Geometry: final body of the model. Coordinates: model frame, mm. Face numbers are marked on the shaded views. A direction names the side the tool comes from. Round coordinates to 2 decimals unless told otherwise and drop trailing zeros. Order: outer loops, then holes, each group sorted by start corner. A loop starts at its lowest first (then second) coordinate and runs counter-clockwise, first axis right, second up. Notation, with made-up numbers: M -31,-36 L 13,-36 A8 ccw 13,-27 Z; hole C 29.5,-2 d3. An arc over 180 degrees is marked long. Put each result on its own line as item: value. Start each with the question number.
1) Material intervals for probe 1 along Y at (x, z) = (-4, -32); probe 2 along Y at (x, z) = (5, 4.5), sorted ascending. Write a range as [from, to].
2) Section B-B, the plane z = 10. Return loops of the section in (x, y).
3) First-contact query: P1, Ø5, axis at y = 25, z = 10, coming from the +X side; P2, Ø12.5, axis at x = -3, y = -3, coming from the +Z side; P3, Ø8, axis at y = -4.5, z = -12.5, coming from the -X side; P4, Ø10, axis at y = 12.5, z = -49, coming from the +X side. Flat tips, straight axial feed; report the tip coordinate or a pass-through.
4) Draft query along Z for the marked faces 1, 2, 3 and 4. Return one class per face: pulls with the +Z half, pulls with the -Z half, needs draft (parallel to the pull), parting line crosses it, or undercut.
5) Section A-A, the plane y = 25. Return loops of the section in (x, z), then the cut area to 3 significant figures.
6) Access query for the marked faces 5 and 6. Directions: +Z, -Z, +X, -X, +Y, -Y. A direction counts if a zero-diameter tool reaches every point of the face in a straight line with its end or side. Return the directions, or none.
from build123d import *

# Parameters (mm, degrees)
EXTRUDE_1_DEPTH          = 5
SKETCH_3_R               = 1.5
EXTRUDE_2_DEPTH          = 4
CUT_EXTRUDE_1_DEPTH      = 112.469065397
PATTERN_CIRCULAR_1_COUNT = 3
FILLET_1_R               = 3
FILLET_2_R               = 5


with BuildPart() as part:
    # 草图1 → 旋转1 (revolve)
    with BuildSketch(Plane(origin=(0, 0, 0), x_dir=(0, 0, -1), z_dir=(1, 0, 0)), mode=Mode.PRIVATE) as revolve_1_sk:
        Polygon((0, 0), (0, 12.5), (3, 12.5), (10.5, 5), (79, 5), (79, 8), (82, 8), (82, 5), (102, 5), (102, 8), (105, 8), (105, 0), align=None)
    revolve(revolve_1_sk.sketch.rotate(Axis((0, 0, 0), (0, 0, -1)), 90), axis=Axis((0, 0, 0), (0, 0, -1)))

    # 草图2 → 凸台-拉伸1 (add)
    with BuildSketch(Plane.XY):
        Polygon((-4, 25), (4, 25), (4, 18.07179677), (17.650635095, -5.57179677), (23.650635095, -9.035898385), (19.650635095, -15.964101615), (13.650635095, -12.5), (-13.650635095, -12.5), (-19.650635095, -15.964101615), (-23.650635095, -9.035898385), (-17.650635095, -5.57179677), (-4, 18.07179677), align=None)
    extrude(amount=EXTRUDE_1_DEPTH)

    # 草图3 → 凸台-拉伸2 (add, symmetric)
    with BuildSketch(Plane(origin=(0, 0, 0), x_dir=(0, 0, -1), z_dir=(1, 0, 0))):
        with BuildLine():
            Line((-5, 7.5), (-13.510549927, 23.082700021))
            ThreePointArc((-13.510549927, 23.082700021), (-12.95059807, 27.700735275), (-8.4, 28.666060556))
            Line((-8.4, 28.666060556), (0, 25))
            Line((0, 25), (-5, 25))
            Line((-5, 25), (-5, 7.5))
        make_face()
        with Locations((-10, 25)):
            Circle(SKETCH_3_R, mode=Mode.SUBTRACT)
    extrude_2 = extrude(amount=EXTRUDE_2_DEPTH, both=True)

    # 草图5 → 切除-拉伸1 (cut, symmetric)
    with BuildSketch(Plane(origin=(0, 0, 0), x_dir=(0, 0, -1), z_dir=(1, 0, 0))):
        Polygon((0, 20), (-6.415605973, 27.8), (0, 25), align=None)
    cut_extrude_1 = extrude(amount=CUT_EXTRUDE_1_DEPTH, both=True, mode=Mode.SUBTRACT)

    # 阵列(圆周)1: 凸台-拉伸2, 切除-拉伸1 ×3 about axis
    pattern_circular_1_axis = Axis((0, 0, 0), (0, 0, 1))
    add([extrude_2.rotate(pattern_circular_1_axis, i * 360 / PATTERN_CIRCULAR_1_COUNT) for i in range(1, PATTERN_CIRCULAR_1_COUNT)])
    add([cut_extrude_1.rotate(pattern_circular_1_axis, i * 360 / PATTERN_CIRCULAR_1_COUNT) for i in range(1, PATTERN_CIRCULAR_1_COUNT)], mode=Mode.SUBTRACT)

    # 圆角1
    # the kernel refuses this fillet: 3 mm, written as the material it adds along each edge
    with BuildSketch(Plane(origin=(20.145825623, -16.25, 5), x_dir=(0, 0, 1), z_dir=(-0.8660254037844384, 0.5000000000000004, 0))) as fillet_1_piece_1_section:
        with BuildLine():
            CenterArc((FILLET_1_R, -FILLET_1_R), FILLET_1_R, 90, 90)
            Line((0, -FILLET_1_R), (0, 0))
            Line((0, 0), (FILLET_1_R, 0))
        make_face()
    fillet_1_piece_1 = extrude(amount=25.57179677, mode=Mode.PRIVATE)
    fillet_1_piece_1 = split(fillet_1_piece_1, bisect_by=Plane(origin=(20.145825623, -12.5, 5), z_dir=(0, 1, 0)), keep=Keep.TOP, mode=Mode.PRIVATE)
    fillet_1_piece_1 = split(fillet_1_piece_1, bisect_by=Plane(origin=(16.550053856, -14.173980202, 12.602327469), z_dir=(0.4151076221534179, -0.23966249739294157, -0.877637481750588)), keep=Keep.TOP, mode=Mode.PRIVATE)
    add(fillet_1_piece_1)
    with BuildSketch(Plane(origin=(24.145825623, -9.32179677, 5), x_dir=(0, 0, 1), z_dir=(-0.8660254037844384, 0.5000000000000004, 0))) as fillet_1_piece_2_section:
        with BuildLine():
            CenterArc((FILLET_1_R, FILLET_1_R), FILLET_1_R, 180, 90)
            Line((0, FILLET_1_R), (0, 0))
            Line((0, 0), (FILLET_1_R, 0))
        make_face()
    fillet_1_piece_2 = extrude(amount=25.57179677, mode=Mode.PRIVATE)
    fillet_1_piece_2 = split(fillet_1_piece_2, bisect_by=Plane(origin=(20.550053856, -7.245776972, 12.602327469), z_dir=(0.4151076221534179, -0.23966249739294157, -0.877637481750588)), keep=Keep.TOP, mode=Mode.PRIVATE)
    fillet_1_piece_2 = split(fillet_1_piece_2, bisect_by=Plane(origin=(20.898230359, -11.19679677, 5), z_dir=(-0.8660254037844386, -0.5000000000000001, 0)), keep=Keep.TOP, mode=Mode.PRIVATE)
    add(fillet_1_piece_2)
    with BuildSketch(Plane(origin=(4, 25.57179677, 5), x_dir=(0, 0, 1), z_dir=(0, -1, 0))) as fillet_1_piece_3_section:
        with BuildLine():
            CenterArc((FILLET_1_R, -FILLET_1_R), FILLET_1_R, 90, 90)
            Line((0, -FILLET_1_R), (0, 0))
            Line((0, 0), (FILLET_1_R, 0))
        make_face()
    fillet_1_piece_3 = extrude(amount=25.57179677, mode=Mode.PRIVATE)
    fillet_1_piece_3 = split(fillet_1_piece_3, bisect_by=Plane(origin=(0.752404736, 23.69679677, 5), z_dir=(-0.8660254037844386, -0.5000000000000001, 0)), keep=Keep.TOP, mode=Mode.PRIVATE)
    fillet_1_piece_3 = split(fillet_1_piece_3, bisect_by=Plane(origin=(4, 21.419757175, 12.602327469), z_dir=(0, 0.4793249947858827, -0.877637481750588)), keep=Keep.TOP, mode=Mode.PRIVATE)
    add(fillet_1_piece_3)
    with BuildSketch(Plane(origin=(-4, 25.57179677, 5), x_dir=(0, 0, 1), z_dir=(0, -1, 0))) as fillet_1_piece_4_section:
        with BuildLine():
            CenterArc((FILLET_1_R, FILLET_1_R), FILLET_1_R, 180, 90)
            Line((0, FILLET_1_R), (0, 0))
            Line((0, 0), (FILLET_1_R, 0))
        make_face()
    fillet_1_piece_4 = extrude(amount=25.57179677, mode=Mode.PRIVATE)
    fillet_1_piece_4 = split(fillet_1_piece_4, bisect_by=Plane(origin=(-0.752404736, 23.69679677, 5), z_dir=(0.8660254037844388, -0.4999999999999999, 0)), keep=Keep.TOP, mode=Mode.PRIVATE)
    fillet_1_piece_4 = split(fillet_1_piece_4, bisect_by=Plane(origin=(-4, 21.419757175, 12.602327469), z_dir=(0, 0.4793249947858827, -0.877637481750588)), keep=Keep.TOP, mode=Mode.PRIVATE)
    add(fillet_1_piece_4)
    with BuildSketch(Plane(origin=(-24.145825623, -9.32179677, 5), x_dir=(0, 0, 1), z_dir=(0.8660254037844388, 0.49999999999999983, 0))) as fillet_1_piece_5_section:
        with BuildLine():
            CenterArc((FILLET_1_R, -FILLET_1_R), FILLET_1_R, 90, 90)
            Line((0, -FILLET_1_R), (0, 0))
            Line((0, 0), (FILLET_1_R, 0))
        make_face()
    fillet_1_piece_5 = extrude(amount=25.57179677, mode=Mode.PRIVATE)
    fillet_1_piece_5 = split(fillet_1_piece_5, bisect_by=Plane(origin=(-20.898230359, -11.19679677, 5), z_dir=(0.8660254037844388, -0.4999999999999999, 0)), keep=Keep.TOP, mode=Mode.PRIVATE)
    fillet_1_piece_5 = split(fillet_1_piece_5, bisect_by=Plane(origin=(-20.550053856, -7.245776972, 12.602327469), z_dir=(-0.4151076221534181, -0.23966249739294126, -0.8776374817505879)), keep=Keep.TOP, mode=Mode.PRIVATE)
    add(fillet_1_piece_5)
    with BuildSketch(Plane(origin=(-20.145825623, -16.25, 5), x_dir=(0, 0, 1), z_dir=(0.8660254037844388, 0.49999999999999983, 0))) as fillet_1_piece_6_section:
        with BuildLine():
            CenterArc((FILLET_1_R, FILLET_1_R), FILLET_1_R, 180, 90)
            Line((0, FILLET_1_R), (0, 0))
            Line((0, 0), (FILLET_1_R, 0))
        make_face()
    fillet_1_piece_6 = extrude(amount=25.57179677, mode=Mode.PRIVATE)
    fillet_1_piece_6 = split(fillet_1_piece_6, bisect_by=Plane(origin=(-20.145825623, -12.5, 5), z_dir=(0, 1, 0)), keep=Keep.TOP, mode=Mode.PRIVATE)
    fillet_1_piece_6 = split(fillet_1_piece_6, bisect_by=Plane(origin=(-16.550053856, -14.173980202, 12.602327469), z_dir=(-0.4151076221534181, -0.23966249739294126, -0.8776374817505879)), keep=Keep.TOP, mode=Mode.PRIVATE)
    add(fillet_1_piece_6)

    # 圆角2
    # the kernel refuses this fillet: 5 mm, written as the material it adds along each edge
    with BuildSketch(Plane(origin=(0, 0, 0), x_dir=(-0.8660253934759007, 0.5000000178549112, 0), z_dir=(-0.5000000178549112, -0.8660253934759007, 0))) as fillet_2_piece_1_section:
        with BuildLine():
            CenterArc((17.082575695, 5), FILLET_2_R, 203.578178478, 66.421821522)
            Line((17.082575695, 0), (12.5, 0))
            Line((12.5, 0), (12.5, 3))
        make_face()
    fillet_2_piece_1 = revolve(axis=Axis((0, 0, 0), (0, 0, -1)), revolution_arc=119.999998782, mode=Mode.PRIVATE)
    fillet_2_piece_1 = split(fillet_2_piece_1, bisect_by=Plane(origin=(-10.825317547, 6.25, 0), z_dir=(0.866025403784329, -0.50000000000019, 0)), keep=Keep.TOP, mode=Mode.PRIVATE)
    fillet_2_piece_1 = split(fillet_2_piece_1, bisect_by=Plane(origin=(10.825317547, 6.25, 0), z_dir=(-0.866025403784329, -0.50000000000019, 0)), keep=Keep.TOP, mode=Mode.PRIVATE)
    add(fillet_2_piece_1)
    with BuildSketch(Plane(origin=(0, 0, 0), x_dir=(3.791753972085742e-09, -1.0, 0), z_dir=(1.0, 3.791753972085742e-09, 0))) as fillet_2_piece_2_section:
        with BuildLine():
            CenterArc((17.082575695, 5), FILLET_2_R, 203.578178478, 66.421821522)
            Line((12.5, 3), (12.5, 0))
            Line((12.5, 0), (17.082575695, 0))
        make_face()
    fillet_2_piece_2 = revolve(axis=Axis((0, 0, 0), (0, 0, -1)), revolution_arc=120.000001399, mode=Mode.PRIVATE)
    fillet_2_piece_2 = split(fillet_2_piece_2, bisect_by=Plane(origin=(-10.825317547, 6.25, 0), z_dir=(0.866025403784329, -0.50000000000019, 0)), keep=Keep.TOP, mode=Mode.PRIVATE)
    fillet_2_piece_2 = split(fillet_2_piece_2, bisect_by=Plane(origin=(0, -12.5, 0), z_dir=(0, 1, 0)), keep=Keep.TOP, mode=Mode.PRIVATE)
    add(fillet_2_piece_2)
    with BuildSketch(Plane(origin=(0, 0, 0), x_dir=(1, 0, 0), z_dir=(0, 1, 0))) as fillet_2_piece_3_section:
        with BuildLine():
            CenterArc((17.082575695, 5), FILLET_2_R, 203.578178478, 66.421821522)
            Line((17.082575695, 0), (12.5, 0))
            Line((12.5, 0), (12.5, 3))
        make_face()
    fillet_2_piece_3 = revolve(axis=Axis((0, 0, 0), (0, 0, -1)), revolution_arc=89.999999783, mode=Mode.PRIVATE)
    fillet_2_piece_3 = split(fillet_2_piece_3, bisect_by=Plane(origin=(10.825317547, 6.25, 0), z_dir=(-0.866025403784329, -0.50000000000019, 0)), keep=Keep.TOP, mode=Mode.PRIVATE)
    fillet_2_piece_3 = split(fillet_2_piece_3, bisect_by=Plane(origin=(0, -12.5, 0), z_dir=(0, 1, 0)), keep=Keep.TOP, mode=Mode.PRIVATE)
    add(fillet_2_piece_3)
    with BuildSketch(Plane(origin=(0, 0, 0), x_dir=(0.8660254034677206, 0.5000000005485719, 0), z_dir=(-0.5000000005485719, 0.8660254034677206, 0))) as fillet_2_piece_4_section:
        with BuildLine():
            CenterArc((17.082575695, 5), FILLET_2_R, 203.578178478, 66.421821522)
            Line((17.082575695, 0), (12.5, 0))
            Line((12.5, 0), (12.5, 3))
        make_face()
    fillet_2_piece_4 = revolve(axis=Axis((0, 0, 0), (0, 0, -1)), revolution_arc=30.000000036, mode=Mode.PRIVATE)
    fillet_2_piece_4 = split(fillet_2_piece_4, bisect_by=Plane(origin=(10.825317547, 6.25, 0), z_dir=(-0.866025403784329, -0.50000000000019, 0)), keep=Keep.TOP, mode=Mode.PRIVATE)
    add(fillet_2_piece_4)
    # the kernel refuses this fillet: 5 mm, written as the material it takes off along each edge
    with BuildSketch(Plane(origin=(-13.080360235, -17.344151491, 0), x_dir=(0.8660254037844387, 0.49999999999999983, 0), z_dir=(-0.49999999999999983, 0.8660254037844388, 0)), Plane(origin=(-8.480295681, 20, 0), x_dir=(0, -1, 0), z_dir=(1, 0, 0))) as fillet_2_2_piece_1:
        with BuildLine():
            CenterArc((FILLET_2_R * 0.358423654455, -FILLET_2_R), FILLET_2_R, 90, 39.437761058)
            Line((-FILLET_2_R * 0.276815994626, -FILLET_2_R * 0.227684916478), (0, 0))
            Line((0, 0), (FILLET_2_R * 0.358423654455, 0))
        make_face()
    extrude(amount=16.960591361, mode=Mode.SUBTRACT)
    with BuildSketch(Plane(origin=(21.560655916, -2.655848509, 0), x_dir=(0.6688444820557844, -0.38615754176090344, 0.6352396490811208), z_dir=(-0.5000000000000004, -0.8660254037844384, 0))) as fillet_2_2_piece_2:
        with BuildLine():
            CenterArc((FILLET_2_R * 0.358423654455, FILLET_2_R), FILLET_2_R, 230.562238942, 39.437761058)
            Line((-FILLET_2_R * 0.276815994626, FILLET_2_R * 0.227684916478), (0, 0))
            Line((0, 0), (FILLET_2_R * 0.358423654455, 0))
        make_face()
    extrude(amount=16.960591361, mode=Mode.SUBTRACT)


solid = part.part
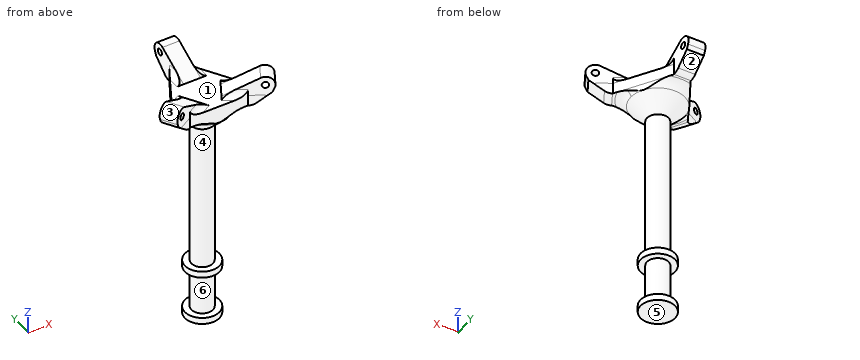
Result sheet:
1. probe 1: y = [-3, 3]
1. probe 2: y = [-12.5, 16.34]
2. outline: M -27.11,-11.04 L -23.11,-17.96 L -20.95,-16.71 L -24.95,-9.79 Z; M -22.35,-8.29 L -18.35,-15.21 L -12.42,-11.79 L -16.42,-4.86 Z; M -4,16.65 L 4,16.65 L 4,23.5 L -4,23.5 Z; M -4,26.5 L 4,26.5 L 4,29 L -4,29 Z; M 12.42,-11.79 L 18.35,-15.21 L 22.35,-8.29 L 16.42,-4.86 Z; M 20.95,-16.71 L 23.11,-17.96 L 27.11,-11.04 L 24.95,-9.79 Z
3. P1: stops at x = 4
3. P2: stops at z = 6.56
3. P3: stops at x = -6
3. P4: passes through
4. face 1: pulls with the +Z half
4. face 2: pulls with the -Z half
4. face 3: parting line crosses it
4. face 4: undercut
5. outline: M -4,4.11 L 4,4.11 L 4,8.5 L -4,8.5 Z; M -4,11.5 L 4,11.5 L 4,14 L -4,14 Z
5. area: 55.1 mm2
6. face 5: -Z, +X, -X, +Y, -Y
6. face 6: none
